```python
from build123d import *

# Parameters (mm, degrees)
SKETCH1_W                     = 85
SKETCH1_H                     = 12
BOSS_EXTRUDE1_DEPTH           = 12
SKETCH2_R                     = 8
CUT_EXTRUDE2_DEPTH            = 5
CUT_EXTRUDE3_START            = -5
SKETCH3_R                     = 8
CUT_EXTRUDE3_DEPTH            = 5
CUT_EXTRUDE4_DEPTH            = 45.567364741
CUT_EXTRUDE4_DEPTH_BACK       = 45.567364741
SKETCH4_R                     = 6
SKETCH5_R                     = 2.625
CUT_EXTRUDE6_DEPTH            = 45.567364741
SKETCH7_R                     = 8.5
BOSS_EXTRUDE3_DEPTH           = 9
BOSS_EXTRUDE3_DRAFT           = 20
BOSS_EXTRUDE3_PROFILE_2_DEPTH = 9
BOSS_EXTRUDE3_PROFILE_2_DRAFT = 20
CHAMFER1_SIZE                 = 1.673157185
CHAMFER1_SIZE_2               = 1
CHAMFER2_SIZE                 = 1
CHAMFER2_SIZE_2               = 1.673157185
CUT_EXTRUDE9_DEPTH            = 4
SKETCH11_R                    = 4.75
CUT_EXTRUDE10_DEPTH           = 51.154760492
SKETCH12_W                    = 84.776225192
SKETCH12_H                    = 9.817436209
CUT_EXTRUDE11_DEPTH           = 52.647846034


with BuildPart() as part:
    # Sketch1 → Boss-Extrude1 (new body)
    with BuildSketch(Plane.XY):
        Rectangle(SKETCH1_W, SKETCH1_H)
    extrude(amount=BOSS_EXTRUDE1_DEPTH)

    # Sketch2 → Cut-Extrude2 (cut)
    with BuildSketch(Plane(origin=(0, 6, 0), x_dir=(1, 0, 0), z_dir=(0, 1, 0))):
        with Locations((-17.5, -12)):
            Circle(SKETCH2_R)
        with Locations((17.5, -12)):
            Circle(SKETCH2_R)
    extrude(amount=-CUT_EXTRUDE2_DEPTH, mode=Mode.SUBTRACT)

    # Sketch3 → Cut-Extrude3 (cut)
    with BuildSketch(Plane.XZ.offset(6).offset(CUT_EXTRUDE3_START)):
        with Locations((-17.5, 12)):
            Circle(SKETCH3_R)
        with Locations((17.5, 12)):
            Circle(SKETCH3_R)
    extrude(amount=CUT_EXTRUDE3_DEPTH, mode=Mode.SUBTRACT)

    # Sketch4 → Cut-Extrude4 (cut, two sides: drawn at the far end of the back side and taken through both)
    with BuildSketch(Plane(origin=(0, 0, 0), x_dir=(1, 0, 0), z_dir=(0, 1, 0)).offset(-CUT_EXTRUDE4_DEPTH_BACK)):
        with Locations((-17.5, -12)):
            Circle(SKETCH4_R)
        with Locations((17.5, -12)):
            Circle(SKETCH4_R)
    extrude(amount=CUT_EXTRUDE4_DEPTH + CUT_EXTRUDE4_DEPTH_BACK, mode=Mode.SUBTRACT)

    # Sketch5 → Cut-Extrude6 (cut, through all)
    with BuildSketch(Plane.XY.offset(12)):
        with Locations((-30, 0)):
            Circle(SKETCH5_R)
        with Locations((30, 0)):
            Circle(SKETCH5_R)
    extrude(amount=-CUT_EXTRUDE6_DEPTH, mode=Mode.SUBTRACT)


with BuildPart() as boss_extrude3_tool:
    # Sketch7 → Boss-Extrude3 (with draft: the straight prism first)
    with BuildSketch(Plane(origin=(0, 6, 0), x_dir=(1, 0, 0), z_dir=(0, 1, 0))):
        with Locations((-17.5, -12)):
            Circle(SKETCH7_R)
    extrude(amount=BOSS_EXTRUDE3_DEPTH)
    # Boss-Extrude3: the draft: its side faces are tilted about the plane it starts from
    boss_extrude3_sides = [boss_extrude3_tool.faces().sort_by_distance(p)[0] for p in [
        (-26, 10.5, 12),
    ]]
    draft(boss_extrude3_sides, Plane(origin=(0, 6, 0), x_dir=(1, 0, 0), z_dir=(0, 1, 0)), BOSS_EXTRUDE3_DRAFT)


with BuildPart() as part_1:
    add(part.part)

    # Boss-Extrude3: add boss_extrude3_tool
    add(boss_extrude3_tool.part)


with BuildPart() as boss_extrude3_profile_2_tool:
    # Sketch7 → Boss-Extrude3 profile 2 (with draft: the straight prism first)
    with BuildSketch(Plane(origin=(0, 6, 0), x_dir=(1, 0, 0), z_dir=(0, 1, 0))):
        with Locations((17.5, -12)):
            Circle(SKETCH7_R)
    extrude(amount=BOSS_EXTRUDE3_PROFILE_2_DEPTH)
    # Boss-Extrude3 profile 2: the draft: its side faces are tilted about the plane it starts from
    boss_extrude3_profile_2_sides = [boss_extrude3_profile_2_tool.faces().sort_by_distance(p)[0] for p in [
        (9, 10.5, 12),
    ]]
    draft(boss_extrude3_profile_2_sides, Plane(origin=(0, 6, 0), x_dir=(1, 0, 0), z_dir=(0, 1, 0)), BOSS_EXTRUDE3_PROFILE_2_DRAFT)


with BuildPart() as part_2:
    add(part_1.part)

    # Boss-Extrude3 profile 2: add boss_extrude3_profile_2_tool
    add(boss_extrude3_profile_2_tool.part)

    # Chamfer1
    # the kernel refuses this chamfer: 1.673157185, 1 mm, written as the material it adds along each edge
    with BuildSketch(Plane(origin=(-17.5, 6, 12), x_dir=(1, 0, 0), z_dir=(0, 0, 1))) as chamfer1_piece_1:
        Polygon((8.5 - CHAMFER1_SIZE * 0.342020143346, CHAMFER1_SIZE * 0.939692620843), (8.5 + CHAMFER1_SIZE_2, 0), (8.5, 0), align=None)
    revolve(axis=Axis((-17.5, 6, 12), (0, 1, 0)), revolution_arc=180)

    # Chamfer2
    # the kernel refuses this chamfer: 1.673157185, 1 mm, written as the material it adds along each edge
    with BuildSketch(Plane(origin=(17.5, 6, 12), x_dir=(1, 0, 0), z_dir=(0, 0, 1))) as chamfer2_piece_1:
        Polygon((8.5 + CHAMFER2_SIZE, 0), (8.5 - CHAMFER2_SIZE_2 * 0.342020143346, CHAMFER2_SIZE_2 * 0.939692620843), (8.5, 0), align=None)
    revolve(axis=Axis((17.5, 6, 12), (0, 1, 0)), revolution_arc=180)

    # Sketch10 → Cut-Extrude9 (cut)
    with BuildSketch(Plane(origin=(0, 15, 0), x_dir=(1, 0, 0), z_dir=(0, 1, 0))):
        Polygon((-17.5, -6.226497308), (-22.5, -9.113248654), (-22.5, -14.886751346), (-17.5, -17.773502692), (-12.5, -14.886751346), (-12.5, -9.113248654), align=None)
        Polygon((17.5, -6.226497308), (12.5, -9.113248654), (12.5, -14.886751346), (17.5, -17.773502692), (22.5, -14.886751346), (22.5, -9.113248654), align=None)
    extrude(amount=-CUT_EXTRUDE9_DEPTH, mode=Mode.SUBTRACT)

    # Sketch11 → Cut-Extrude10 (cut, through all)
    with BuildSketch(Plane(origin=(0, 11, 0), x_dir=(1, 0, 0), z_dir=(0, 1, 0))):
        with Locations((-17.5, -12)):
            Circle(SKETCH11_R)
        with Locations((17.5, -12)):
            Circle(SKETCH11_R)
    extrude(amount=-CUT_EXTRUDE10_DEPTH, mode=Mode.SUBTRACT)

    # Sketch12 → Cut-Extrude11 (cut, through all)
    with BuildSketch(Plane.XZ.offset(6)):
        with Locations((-0.111887404, 16.908718105)):
            Rectangle(SKETCH12_W, SKETCH12_H)
    extrude(amount=-CUT_EXTRUDE11_DEPTH, mode=Mode.SUBTRACT)


solid = part_2.part
```
Verification items for the finished model (mm, model axes). A direction names the side the tool comes from. Coordinates: 2 decimals unless noted, no trailing zeros. Order: outer loops, then holes, each group sorted by start corner. A loop starts at its lowest first (then second) coordinate and runs counter-clockwise, first axis right, second up. Notation, with made-up numbers: (83, -33) -> (92, -33) arc R19 ccw to (92, -11) -> close; hole circle Ø10 at (52, 36). An arc over 180 degrees is marked (long way). Put each result on its own line as item: value. Start each with the question number.
1) Cross-section at B-B (x = -30). Enter the section's corners in (y, z) (3 decimals).
2) Tool access check on faces 1 (the cylindrical face through (-17.324, 3.535, 4.002)), 2 (the flat face through (16, -1, 6)), 3 (the flat face through (20.035, 13.028, 7.69)). Record the directions out of +Z, -Z, +X, -X, +Y, -Y that give a thin tool (end or side, any length) a straight path to the whole face; none if there is none.
3) Material ranges on L1, parallel to Y at x = 30, z = 6 (3 decimals); L2, parallel to X at y = 12.5, z = 11.5; L3, parallel to X at y = 0.5, z = 9.75, recorded low to high.
4) Go/stop test with flat-tipped pins: pin 1 (2.5 mm diameter, centred on y = 14, z = 10.5, fed in from +X); pin 2 (0.9 mm diameter, centred on y = 12, z = 10, fed in from -X); pin 3 (1.5 mm diameter, centred on x = -8, z = 4.5, fed in from +Y). Record where each tip stops, or that it passes through.
5) Release check for a two-part mould opening along Y. For faces 4 (the cylindrical face through (17.6, 8.54, 7.25)), 5 (the flat face through (-19, -1, 6)), 6 (the cylindrical face through (-32.622, 0.115, 6.084)) record: pulls with the +Y half, pulls with the -Y half, needs draft (parallel to the pull), parting line crosses it, or undercut.
6) Cross-section at A-A (y = 0). Enter the section's corners in (x, z) (3 decimals).
Geometry check:
1. outline: (-6, 0) -> (-2.625, 0) -> (-2.625, 12) -> (-6, 12) -> close; (2.625, 0) -> (6, 0) -> (6, 12) -> (2.625, 12) -> close
2. face 1: +Z
2. face 2: +Z, -Y
2. face 3: +Z, +Y
3. L1: y = -6 to -2.625, 2.625 to 6
3. L2: x = -23.61 to -22.5, -12.5 to -11.39, 11.39 to 12.5, 22.5 to 23.61
3. L3: x = -42.5 to -32.58, -27.42 to -23.06, -11.94 to 11.94, 23.06 to 27.42, 32.58 to 42.5
4. pin 1: stops at x = 23.42
4. pin 2: stops at x = -23.71
4. pin 3: stops at y = 6
5. face 4: needs draft
5. face 5: pulls with the -Y half
5. face 6: undercut
6. outline: (-42.5, 0) -> (-32.625, 0) -> (-32.625, 12) -> (-42.5, 12) -> close; (-27.375, 0) -> (27.375, 0) -> (27.375, 12) -> (23.5, 12) arc R6 cw to (11.5, 12) -> (-11.5, 12) arc R6 cw to (-23.5, 12) -> (-27.375, 12) -> close; (32.625, 0) -> (42.5, 0) -> (42.5, 12) -> (32.625, 12) -> close
